from build123d import *

# Parameters (mm, degrees)
F0_W     = 76.2
F0_H     = 25.4
F1_DEPTH = 19.05
F3_DEPTH = 76.2
F4_DEPTH = 76.2
F6_DEPTH = 76.2


with BuildPart() as f1:
    # F0 (on Top) → F1 (new body)
    with BuildSketch(Plane.XY):
        with Locations((0.7800040767, 0.3926137724)):
            Rectangle(F0_W, F0_H)
    extrude(amount=F1_DEPTH)

    # F2 (on face) → F3 (cut)
    with BuildSketch(Plane(origin=(-37.3199959233, 0, 0), x_dir=(0, -1, 0), z_dir=(-1, 0, 0))):
        Polygon((5.1924203255, 19.05), (-4.8661371025, 19.05), (-8.724951177, 7.6794241368), (0.294794015, 4.6184076928), align=None)
    extrude(amount=-F3_DEPTH, mode=Mode.SUBTRACT)

    # F2 (on face) → F4 (cut)
    with BuildSketch(Plane(origin=(-37.3199959233, 0, 0), x_dir=(0, -1, 0), z_dir=(-1, 0, 0))):
        Polygon((-13.0926137724, 3.9323569939), (-7.9621635377, 19.05), (-13.0926137724, 19.05), align=None)
    extrude(amount=-F4_DEPTH, mode=Mode.SUBTRACT)

    # F5 (on face) → F6 (cut)
    with BuildSketch(Plane(origin=(-37.3199959233, 0, 0), x_dir=(0, -1, 0), z_dir=(-1, 0, 0))):
        Polygon((12.3073862276, 19.05), (8.7499032765, 19.05), (3.2798947146, 2.9317973285), (8.4929587319, 2.9317973285), (12.3073862276, 2.9317973285), align=None)
    extrude(amount=-F6_DEPTH, mode=Mode.SUBTRACT)


solid = f1.part
The model under review builds one solid part; all positions refer to its coordinate system, in mm. A direction names the side the tool comes from. Give positions to 0.01 mm unless a question says otherwise; leave off trailing zeros. Write each loop counter-clockwise with the first axis right and the second up, starting at its lowest first coordinate (ties: lowest second). Pieces come first, ordered by that corner, then holes. Notation, with made-up numbers: M -3.5,54.5 L 21.5,54.5 A20 ccw 21.5,72.5 Z; hole C 79,11.25 d6. An arc over 180 degrees is marked long. One line per question, with ' | ' between items. Start each with the question number.
Item 1: We need section D-D on y = 1. Write out the cut boundary in (x, z).
Item 2: We need section A-A on y = -6.75. Write out the cut boundary in (x, z).
Item 3: For faces 1 (the flat face through (0, 6, 19.05)), 2 (the flat face through (0.25, 4.28, 6.17)), 3 (the flat face through (0.2, -2.7, 11.7)), 4 (the flat face through (0.25, -6.05, 11.1)), 5 (the flat face through (0.25, 10.56, 11.39)), list the 3-axis set-ups (+Z, -Z, +X, -X, +Y, -Y) from which the entire face can be reached by the end or side of a thin tool; tool diameter is ignored.
Item 4: We need section C-C on z = 8.75. Write out the cut boundary in (x, y), plus the area to 3 significant figures.
Item 5: We need section B-B on x = 17.5. Write out the cut boundary in (y, z), plus the area to 3 significant figures.
Item 6: Wall thickness on line 1 (Y direction, x = 33.5, z = 10.75); line 2 (Y direction, x = -26, z = 8.25); line 3 (Z direction, x = 29.5, y = 2.5): over which ranges is each line inside the solid? List them lowest first. Write a range as from..to.
Item 7: For pin 1 (2 mm diameter, centred on y = 4, z = 16, fed in from -X); pin 2 (10 mm diameter, centred on x = 15, z = 12.5, fed in from +Y); pin 3 (2 mm diameter, centred on x = 23, z = 16.5, fed in from +Y); pin 4 (10 mm diameter, centred on x = -6, z = 8, fed in from -Y), all flat-tipped, find the tip position at first contact; note any pin that passes through.
Item 8: Draft analysis for pull direction Z (two halves, no side actions). For faces 6 (the flat face through (0, -8, 2.932)), 7 (the flat face through (0, 1, 0)), 8 (the flat face through (0, 13.093, 2)), state which applies: released by +Z, released by -Z, zero draft, split by the parting line, or undercut.
Results found:
1) outline: M -37.32,0 L 38.88,0 L 38.88,5.06 L -37.32,5.06 Z
2) outline: M -37.32,0 L 38.88,0 L 38.88,2.93 L -37.32,2.93 Z; M -37.32,13.16 L 38.88,13.16 L 38.88,19.05 L -37.32,19.05 Z
3) face 1: +Z, +X, -X, +Y, -Y | face 2: +X, -X | face 3: +Z, +X, -X | face 4: +X, -X, -Y | face 5: +Z, +X, -X, +Y
4) outline: M -37.32,-5.25 L 38.88,-5.25 L 38.88,-1.7 L -37.32,-1.7 Z; M -37.32,8.36 L 38.88,8.36 L 38.88,11.46 L -37.32,11.46 Z | area: 507 mm2
5) outline: M -12.31,0 L 13.09,0 L 13.09,3.93 L 7.96,19.05 L 4.87,19.05 L 8.72,7.68 L -0.29,4.62 L -5.19,19.05 L -8.75,19.05 L -3.28,2.93 L -12.31,2.93 Z | area: 214 mm2
6) line 1: y = -5.93..-2.38, 7.68..10.78 | line 2: y = -5.08..-1.53, 8.53..11.63 | line 3: z = 0..5.57
7) pin 1: passes through | pin 2: stops at y = 11.88 | pin 3: stops at y = 9.17 | pin 4: stops at y = -6.7
8) face 6: undercut | face 7: released by -Z | face 8: zero draft
